Here's the drawing with two shaded views (mm, measured from the low corner). I have some questions. A direction names the side the tool comes from. Coordinates: 2 decimals unless noted, no trailing zeros. Write each loop counter-clockwise with the first axis right and the second up, starting at its lowest first coordinate (ties: lowest second). Pieces come first, ordered by that corner, then holes.
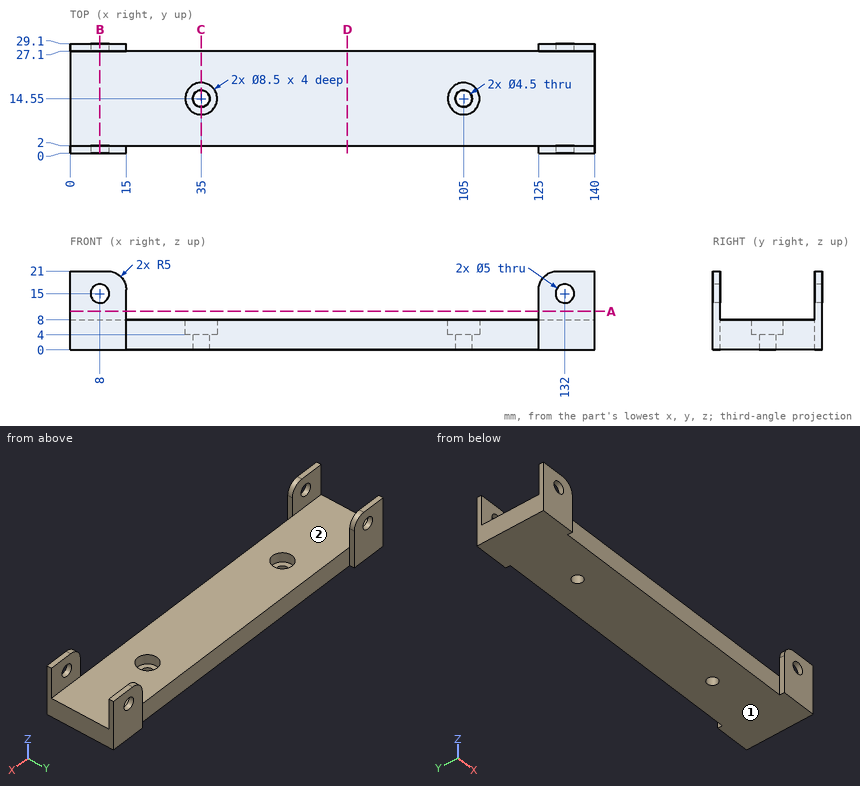
1. If we section it at C-C, the plane x = 35: List the corners of the cut face in (y, z) for me, plus the area to 3 significant figures.
2. If we section it at B-B, the plane x = 8: List the corners of the cut face in (y, z) for me.
3. Which directions (+Z, -Z, +X, -X, +Y, -Y) give clear straight access to the entire face, cutting with the end or side of a thin tool? Please do the marked faces 1 and 2.
4. If we section it at D-D, the plane x = 74: List the corners of the cut face in (y, z) for me, plus the area to 3 significant figures.
5. I'm going to push flat-ended pins straight in: P1, Ø4.5, axis at x = 8, z = 15, coming from the +Y side; P2, Ø2.5, axis at x = 37, y = 14.5, coming from the +Z side; P3, Ø6, axis at x = 71.5, z = 6.5, coming from the +Y side; P4, Ø7.5, axis at x = 98.5, y = 14.5, coming from the +Z side. Where does each tip first touch, or does it pass through?
6. If I drill on L1, parallel to Z at x = 8, y = 1; L2, parallel to X at y = 14.55, z = 1; L3, parallel to Z at x = 22.5, y = 11.5, over which ranges is the centre line in solid material (lowest first)?
7. If we section it at A-A, the plane z = 10.25: List the corners of the cut face in (x, y) for me, plus the area to 3 significant figures.
Answers:
1. outline: (2, 0) - (12.3, 0) - (12.3, 4) - (10.3, 4) - (10.3, 8) - (2, 8) - close; (16.8, 0) - (27.1, 0) - (27.1, 8) - (18.8, 8) - (18.8, 4) - (16.8, 4) - close
1. area: 149 mm2
2. outline: (0, 0) - (29.1, 0) - (29.1, 12.5) - (27.1, 12.5) - (27.1, 8) - (2, 8) - (2, 12.5) - (0, 12.5) - close; (0, 17.5) - (2, 17.5) - (2, 21) - (0, 21) - close; (27.1, 17.5) - (29.1, 17.5) - (29.1, 21) - (27.1, 21) - close
3. face 1: -Z, +X, -X, +Y, -Y
3. face 2: +Z, +X, -X
4. outline: (2, 0) - (27.1, 0) - (27.1, 8) - (2, 8) - close
4. area: 201 mm2
5. P1: passes through
5. P2: stops at z = 4
5. P3: stops at y = 27.1
5. P4: stops at z = 8
6. L1: z = 0 to 12.5, 17.5 to 21
6. L2: x = 0 to 32.75, 37.25 to 102.75, 107.25 to 140
6. L3: z = 0 to 8
7. outline: (0, 0) - (15, 0) - (15, 2) - (0, 2) - close; (0, 27.1) - (15, 27.1) - (15, 29.1) - (0, 29.1) - close; (125, 0) - (140, 0) - (140, 2) - (125, 2) - close; (125, 27.1) - (140, 27.1) - (140, 29.1) - (125, 29.1) - close
7. area: 120 mm2
